Design review of the part built by this model. Coordinates are the model's own, in mm. A direction names the side the tool comes from. Round coordinates to 2 decimals unless told otherwise and drop trailing zeros. Order: outer loops, then holes, each group sorted by start corner. A loop starts at its lowest first (then second) coordinate and runs counter-clockwise, first axis right, second up.
from build123d import *

# Parameters (mm, degrees)
F1_DEPTH = 19.05


with BuildPart() as f1:
    # F0 (on Top) → F1 (new body)
    with BuildSketch(Plane.XY):
        with BuildLine():
            Line((-30.586306, 0), (4.838097, 0))
            Line((4.838097, 0), (54.538528, 0))
            Line((54.538528, 0), (54.538528, 106.68))
            Line((54.538528, 106.68), (-47.061472, 81.28))
            ThreePointArc((-47.061472, 81.28), (-26.797886, 43.077628), (-30.586306, 0))
        make_face()
        with BuildLine():
            Line((54.538528, 0), (4.838097, 0))
            Line((4.838097, 0), (-30.586306, 0))
            ThreePointArc((-30.586306, 0), (-32.021192, -3.397376), (-33.618778, -6.721347))
            Line((-33.618778, -6.721347), (54.538528, -50.8))
            Line((54.538528, -50.8), (54.538528, 0))
        make_face()
        with BuildLine():
            Line((54.538528, -50.8), (-33.618778, -6.721347))
            ThreePointArc((-33.618778, -6.721347), (-39.630922, -16.571075), (-47.061472, -25.4))
            Line((-47.061472, -25.4), (54.538528, -50.8))
        make_face()
        with BuildLine():
            Line((54.538528, 106.68), (54.538528, 0))
            Line((54.538528, 0), (54.538528, -50.8))
            ThreePointArc((54.538528, -50.8), (76.455684, 27.94), (54.538528, 106.68))
        make_face()
    extrude(amount=F1_DEPTH)


solid = f1.part
1) To check wall thickness, follow line 1 along Y through (x, z) = (-39, 8); line 2 along Y through (x, z) = (-33.5, 6.25); line 3 along Y through (x, z) = (63, 9.75). State the ranges of each line that lie inside material, in increasing order.
Results:
line 1: y = -27.42 to -15.68, 71.56 to 83.3
line 2: y = -28.79 to -6.49, 62.37 to 84.67
line 3: y = -34.67 to 90.55
2) Take a section at C-C on x = 69. Give the boundary of the cut face in (y, z), plus the area to 3 significant figures.
Results:
outline: (-19.14, 0) - (75.02, 0) - (75.02, 19.05) - (-19.14, 19.05) - close
area: 1,790 mm2
3) For faces 4 (the face through (-32, -3.35, 9.39)), 5 (the face through (14, 29, 19.05)), list the 3-axis set-ups (+Z, -Z, +X, -X, +Y, -Y) from which the entire face can be reached by the end or side of a thin tool; tool diameter is ignored.
Results:
face 4: +Z, -Z, -X
face 5: +Z, +X, -X, +Y, -Y
4) Clearance check with flat-ended pins moving along their axes: P1, Ø1, axis at y = 8, z = 5, coming from the -X side; P2, Ø10, axis at y = 58, z = 4, coming from the +X side; P3, Ø6, axis at x = 5, z = 13.5, coming from the +Y side. State where each tip first meets the part, or that it passes through.
Results:
P1: stops at x = -28.07
P2: stops at x = 74.38
P3: stops at y = 95.05
5) Take a section at A-A on z = 9.75. Give the boundary of the cut face in (x, y), plus the area to 3 significant figures.
Results:
outline: (-47.06, -25.4) - (54.54, -50.8) arc R152.4 ccw to (54.54, 106.68) - (-47.06, 81.28) arc R76.2 cw to (-30.59, 0) arc R76.2 cw to (-33.62, -6.72) arc R76.2 cw to start
area: 14,200 mm2
6) Take a section at B-B on y = 7.5. Give the boundary of the cut face in (x, z), plus the area to 3 significant figures.
Results:
outline: (-28.07, 0) - (75.08, 0) - (75.08, 19.05) - (-28.07, 19.05) - close
area: 1,970 mm2
7) The part is to be moulded in two halves that separate along Y. For faces 1 (the face through (-26.922, 43.679, 9.392)), 2 (the face through (76.45, 26.78, 9.39)), 3 (the face through (4.45, 94.158, 9.392)), say which applies: released by +Y, released by -Y, zero draft, split by the parting line, or undercut.
Results:
face 1: undercut
face 2: split by the parting line
face 3: released by +Y
